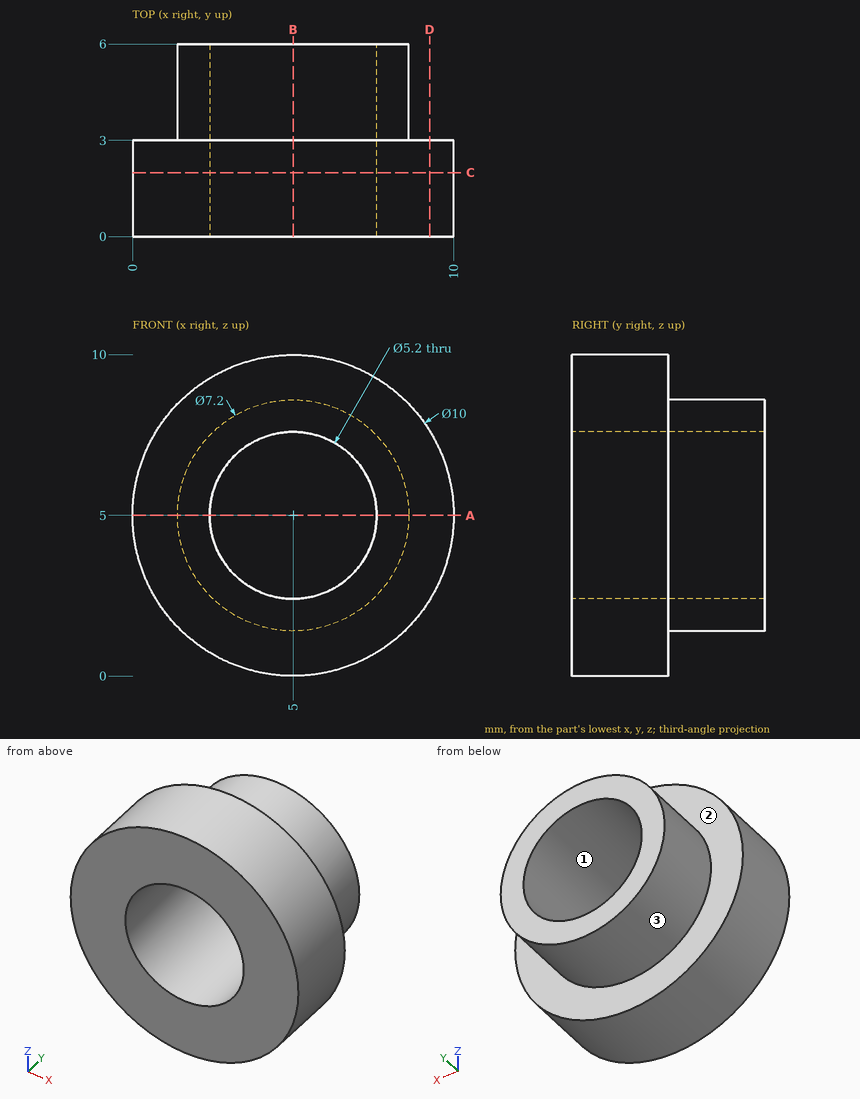
Geometry check sheet. Reference: drawing and pictorial views, mm from the part's lowest x, y, z. Coordinates: 2 decimals unless noted, no trailing zeros. Write each loop counter-clockwise with the first axis right and the second up, starting at its lowest first coordinate (ties: lowest second). Pieces come first, ordered by that corner, then holes.
Item 1: Scan lines: probe 1 along X at (y, z) = (2.15, 5); probe 2 along Z at (x, y) = (5, 4.25). Record each from-to range of solid material in increasing order.
Numbers:
probe 1: x = 0 to 2.4, 7.6 to 10
probe 2: z = 1.4 to 2.4, 7.6 to 8.6
Item 2: Cross-section at A-A on z = 5. Record the boundary of the cut face in (x, y).
Numbers:
outline: (0, 0) - (2.4, 0) - (2.4, 6) - (1.4, 6) - (1.4, 3) - (0, 3) - close; (7.6, 0) - (10, 0) - (10, 3) - (8.6, 3) - (8.6, 6) - (7.6, 6) - close
Item 3: Cross-section at D-D on x = 9.25. Record the boundary of the cut face in (y, z), then the cut area to 3 significant figures.
Numbers:
outline: (0, 2.37) - (3, 2.37) - (3, 7.63) - (0, 7.63) - close
area: 15.8 mm2
Item 4: Mould release check, pull along Z, two halves, no side actions. Record for the marked faces 1, 2 and 3: released by +Z, released by -Z, zero draft, split by the parting line, or undercut.
Numbers:
face 1: undercut
face 2: zero draft
face 3: split by the parting line
Item 5: Cross-section at B-B on x = 5. Record the boundary of the cut face in (y, z).
Numbers:
outline: (0, 0) - (3, 0) - (3, 1.4) - (6, 1.4) - (6, 2.4) - (0, 2.4) - close; (0, 7.6) - (6, 7.6) - (6, 8.6) - (3, 8.6) - (3, 10) - (0, 10) - close
Item 6: Cross-section at C-C on y = 2. Record the boundary of the cut face in (x, z), then the cut area to 3 significant figures.
Numbers:
outline: circle Ø10 at (5, 5); hole circle Ø5.2 at (5, 5)
area: 57.3 mm2
Item 7: Depth check by flat-ended pin: pin 1 Ø1 at (x, z) = (3, 6) entering from +Y; pin 2 Ø1 at (x, y) = (7, 3) entering from -Z. Enter the tip coordinate at first touch or a pass-through.
Numbers:
pin 1: stops at y = 6
pin 2: stops at z = 0.23
